Build history of the part. All positions in model axes, mm. Give positions to 0.01 mm unless a question says otherwise; leave off trailing zeros. Order: outer loops, then holes, each group sorted by start corner. A loop starts at its lowest first (then second) coordinate and runs counter-clockwise, first axis right, second up. Notation, with made-up numbers: M 50,14 L 66,14 A25 cw 66,41 Z; hole C 13,-13 d6. An arc over 180 degrees is marked long. One line per item, written item: value.
from build123d import *

# Parameters (mm, degrees)
F0_W     = 80.1909789443
F0_H     = 62.0844513178
F1_DEPTH = 76.2
F1_TAPER = -3
F2_R     = 29.8619780209
F3_DEPTH = 76.2
F3_TAPER = -3


with BuildPart() as f1:
    # F0 (on Front) → F1 (new body)
    with BuildSketch(Plane.XZ):
        with Locations((17.5543613732, 1.1086538434)):
            Rectangle(F0_W, F0_H)
    extrude(amount=F1_DEPTH, taper=F1_TAPER)

    # F2 (on face) → F3 (join)
    with BuildSketch(Plane.XZ.offset(76.2)):
        with Locations((31.7813456059, 36.1443522837)):
            Circle(F2_R)
    extrude(amount=F3_DEPTH, taper=F3_TAPER)


solid = f1.part
1) Saw through at A-A, the plane y = -98. Write the cut outline in (x, z), then the cut area to 3 significant figures.
Check values:
outline: C 31.78,36.14 d62.01
area: 3,020 mm^2
2) Drill centre lines: probe 1 along Y at (x, z) = (-13, 21); probe 2 along Y at (x, z) = (16.5, 55.5); probe 3 along Z at (x, y) = (11.5, -106.5). Where is each one in solid material? Low to high. Write a range as from..to.
Check values:
probe 1: -76.2..0
probe 2: -152.4..-76.2
probe 3: 12.11..60.18
3) Mould opens along Y. For faces 1 (the face through (31, -152.4, 37)), 2 (the face through (17, 0, 1)), 3 (the face through (6.48, -114.83, 16.74)) say: released by +Y, released by -Y, zero draft, split by the parting line, or undercut.
Check values:
face 1: released by -Y
face 2: released by +Y
face 3: undercut
4) Pin check, flat tips, straight feed: pin 1 (12 mm diameter, centred on x = -6.5, z = 12.5, fed in from -Y); pin 2 (12 mm diameter, centred on x = 16, z = 30.5, fed in from +Y); pin 3 (2 mm diameter, centred on y = -135, z = 31.5, fed in from +X); pin 4 (2 mm diameter, centred on x = 26, y = -24.5, fed in from +Z). Stop position of each tip, or through.
Check values:
pin 1: y = -76.2
pin 2: y = 0
pin 3: x = 64.53
pin 4: z = 33.49
